Geometry: see drawing. Coordinates: mm, zero at the bounding-box minimum. Give positions to 0.01 mm unless a question says otherwise; leave off trailing zeros. Loops run counter-clockwise (first coordinate to the right, second up) from the corner with the lowest first, then second, coordinate; pieces in that order, holes last. Notation, with made-up numbers: (3, -5.75) -> (19, -5.75) arc R28 ccw to (19, 24.25) -> close; hole circle Ø6 at (-9.5, 36.5). An arc over 180 degrees is marked (long way). Answer in a Markdown table with one row per item. Add a question column.
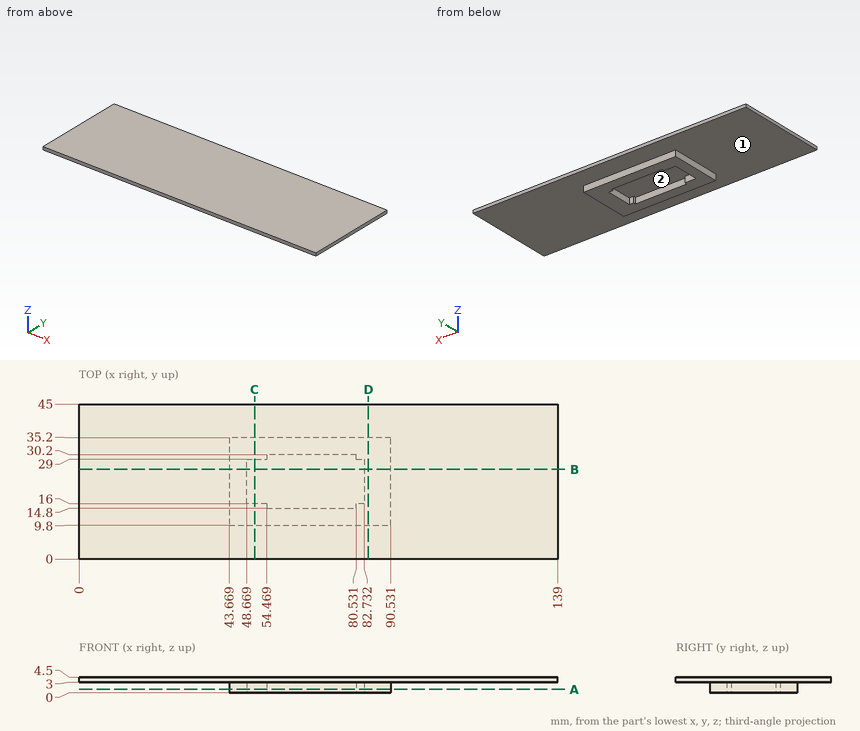
1) Section B-B on y = 26. Output: boundary loops of the cut face in (x, z).
2) Section D-D on x = 84. Output: boundary loops of the cut face in (y, z), and give its area (3 significant figures).
3) Section C-C on x = 51. Output: boundary loops of the cut face in (y, z), and give its area (3 significant figures).
4) Material intervals for line 1 along Y through (x, z) = (75.5, 0.2); line 2 along X through (y, z) = (18.5, 0.2); line 3 along Z through (x, y) = (129, 22.5), sorted ascending.
5) Pin query (flat end, axial travel): pin 1 (2.5 mm diameter, centred on x = 51, z = 1, fed in from -Y); pin 2 (0.9 mm diameter, centred on y = 23, z = 2, fed in from -X); pin 3 (1 mm diameter, centred on y = 30, z = 2, fed in from +X); pin 4 (1.5 mm diameter, centred on x = 23, z = 1.5, fed in from +Y). Return the tip coordinate at first contact, or that it passes through.
6) Section A-A on z = 0.95. Output: boundary loops of the cut face in (x, y).
7) Pull-direction query (Y, two-part tool) for the marked faces 1 and 2; classes: +Y half, -Y half, draft (parallel to the pull), parting line (faces both ways), or undercut.
Working result:
| question | item | result |
|---|---|---|
| 1 | outline | (0, 3) -> (43.67, 3) -> (43.67, 0) -> (48.67, 0) -> (48.67, 3) -> (82.73, 3) -> (82.73, 0) -> (90.53, 0) -> (90.53, 3) -> (139, 3) -> (139, 4.5) -> (0, 4.5) -> close |
| 2 | outline | (0, 3) -> (9.8, 3) -> (9.8, 0) -> (35.2, 0) -> (35.2, 3) -> (45, 3) -> (45, 4.5) -> (0, 4.5) -> close |
| 2 | area | 144 mm2 |
| 3 | outline | (0, 3) -> (9.8, 3) -> (9.8, 0) -> (16, 0) -> (16, 3) -> (29, 3) -> (29, 0) -> (35.2, 0) -> (35.2, 3) -> (45, 3) -> (45, 4.5) -> (0, 4.5) -> close |
| 3 | area | 105 mm2 |
| 4 | line 1 | y = 9.8 to 14.8, 30.2 to 35.2 |
| 4 | line 2 | x = 43.67 to 48.67, 82.73 to 90.53 |
| 4 | line 3 | z = 3 to 4.5 |
| 5 | pin 1 | stops at y = 9.8 |
| 5 | pin 2 | stops at x = 43.67 |
| 5 | pin 3 | stops at x = 90.53 |
| 5 | pin 4 | passes through |
| 6 | outline | (43.67, 9.8) -> (90.53, 9.8) -> (90.53, 35.2) -> (43.67, 35.2) -> close; hole (48.67, 16) -> (54.47, 16) -> (54.47, 14.8) -> (80.53, 14.8) -> (80.53, 16) -> (82.73, 16) -> (82.73, 29) -> (80.53, 29) -> (80.53, 30.2) -> (54.47, 30.2) -> (54.47, 29) -> (48.67, 29) -> close |
| 7 | face 1 | draft |
| 7 | face 2 | undercut |
